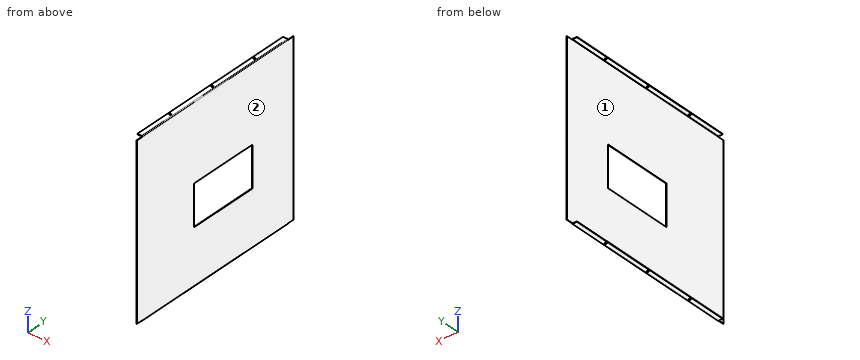
```python
from build123d import *

# Parameters (mm, degrees)
SKETCH_1_W                       = 1.5
SKETCH_1_H                       = 560.17
SM_BASE_FLANGE_1_DEPTH           = 500
SKETCH_6_W                       = 317.570371398
SKETCH_6_H                       = 336.908787646
CUT_EXTRUDE_1_DEPTH              = 10
SKETCH_7_W                       = 1.5
SKETCH_7_H                       = 317.570371398
EXTRUDE_1_DEPTH                  = 34.77
SKETCH_8_W                       = 1.5
SKETCH_8_H                       = 317.570371398
EXTRUDE_2_DEPTH                  = 92.14
SKETCH_9_W                       = 1.5
SKETCH_9_H                       = 209.998787646
EXTRUDE_3_DEPTH                  = 126
SKETCH_10_W                      = 1.5
SKETCH_10_H                      = 209.998787646
EXTRUDE_4_DEPTH                  = 73
SM_EDGE_FLANGE_1_STRIP_W         = 7.4732
SM_EDGE_FLANGE_1_STRIP_H         = 1.5
SM_EDGE_FLANGE_1_STRIP_CUT_DEPTH = 560.17
SM_EDGE_FLANGE_1_DEPTH           = 560.17
SM_EDGE_FLANGE_2_STRIP_W         = 7.4732
SM_EDGE_FLANGE_2_STRIP_H         = 1.5
SM_EDGE_FLANGE_2_STRIP_CUT_DEPTH = 560.17
SM_EDGE_FLANGE_2_DEPTH           = 560.17
SKETCH_19_W                      = 22.446307896
SKETCH_19_H                      = 4.345643328
SKETCH_19_H_2                    = 10.457116237
CUT_EXTRUDE_2_DEPTH              = 20
SKETCH_20_W                      = 19.209439619
SKETCH_20_H                      = 11.495536561
SKETCH_20_W_2                    = 27.208670792
SKETCH_20_H_2                    = 7.195465163
CUT_EXTRUDE_3_DEPTH              = 20
SKETCH_21_R                      = 2.75
CUT_EXTRUDE_4_DEPTH              = 20
CUT_EXTRUDE_START                = -10
SKETCH_22_R                      = 2.75
CUT_EXTRUDE_5_DEPTH              = 10


# Sheet-metal steps are written as plain solids
with BuildPart() as part:
    # Sketch 1 → 基体-法兰1 (new body)
    with BuildSketch(Plane.XY):
        with Locations((0.75, 280.085)):
            Rectangle(SKETCH_1_W, SKETCH_1_H)
    extrude(amount=SM_BASE_FLANGE_1_DEPTH)

    # 草图6 → 切除-拉伸1 (cut)
    with BuildSketch(Plane(origin=(1.5, 0, 0), x_dir=(0, 0, -1), z_dir=(1, 0, 0))):
        with Locations((-246.249491055, 280.085)):
            Rectangle(SKETCH_6_W, SKETCH_6_H)
    extrude(amount=-CUT_EXTRUDE_1_DEPTH, mode=Mode.SUBTRACT)

    # 草图7 → 凸台-拉伸1 (add)
    with BuildSketch(Plane.XZ.offset(-448.539393823)):
        with Locations((0.75, 246.249491055)):
            Rectangle(SKETCH_7_W, SKETCH_7_H)
    extrude(amount=EXTRUDE_1_DEPTH)

    # 草图8 → 凸台-拉伸2 (add)
    with BuildSketch(Plane(origin=(0, 111.630606177, 0), x_dir=(1, 0, 0), z_dir=(0, 1, 0))):
        with Locations((0.75, -246.249491055)):
            Rectangle(SKETCH_8_W, SKETCH_8_H)
    extrude(amount=EXTRUDE_2_DEPTH)

    # 草图9 → 凸台-拉伸3 (add)
    with BuildSketch(Plane(origin=(0, 0, 405.034676754), x_dir=(-1, 0, 0), z_dir=(0, 0, -1))):
        with Locations((-0.75, 308.77)):
            Rectangle(SKETCH_9_W, SKETCH_9_H)
    extrude(amount=EXTRUDE_3_DEPTH)

    # 草图10 → 凸台-拉伸4 (add)
    with BuildSketch(Plane.XY.offset(87.464305356)):
        with Locations((0.75, 308.77)):
            Rectangle(SKETCH_10_W, SKETCH_10_H)
    extrude(amount=EXTRUDE_4_DEPTH)

    # 边线-法兰1 strip (across the edge) → 边线-法兰1 strip cut (cut)
    with BuildSketch(Plane(origin=(0, 0, 500), x_dir=(0, 0, -1), z_dir=(0, 1, 0))):
        with Locations((-1.5, -0.75)):
            Rectangle(SM_EDGE_FLANGE_1_STRIP_W, SM_EDGE_FLANGE_1_STRIP_H)
    extrude(amount=SM_EDGE_FLANGE_1_STRIP_CUT_DEPTH, mode=Mode.SUBTRACT)

    # 边线-法兰1 section (across the edge) → 边线-法兰1 (add)
    with BuildSketch(Plane(origin=(0, 0, 500), x_dir=(0, 0, -1), z_dir=(0, 1, 0))):
        with BuildLine():
            Line((0, 0.7366), (0, 13.5))
            Line((0, 13.5), (1.5, 13.5))
            Line((1.5, 13.5), (1.5, 0.7366))
            ThreePointArc((1.5, 0.7366), (1.715745145, 0.215745145), (2.2366, 0))
            Line((2.2366, 0), (2.2366, -1.5))
            ThreePointArc((2.2366, -1.5), (0.655084973, -0.844915027), (0, 0.7366))
        make_face()
    extrude(amount=SM_EDGE_FLANGE_1_DEPTH)

    # 边线-法兰2 strip (across the edge) → 边线-法兰2 strip cut (cut)
    with BuildSketch(Plane(origin=(0, 560.17, 0), x_dir=(0, 0, 1), z_dir=(0, -1, 0))):
        with Locations((-1.5, -0.75)):
            Rectangle(SM_EDGE_FLANGE_2_STRIP_W, SM_EDGE_FLANGE_2_STRIP_H)
    extrude(amount=SM_EDGE_FLANGE_2_STRIP_CUT_DEPTH, mode=Mode.SUBTRACT)

    # 边线-法兰2 section (across the edge) → 边线-法兰2 (add)
    with BuildSketch(Plane(origin=(0, 560.17, 0), x_dir=(0, 0, 1), z_dir=(0, -1, 0))):
        with BuildLine():
            Line((0, 0.7366), (0, 13.5))
            Line((0, 13.5), (1.5, 13.5))
            Line((1.5, 13.5), (1.5, 0.7366))
            ThreePointArc((1.5, 0.7366), (1.715745145, 0.215745145), (2.2366, 0))
            Line((2.2366, 0), (2.2366, -1.5))
            ThreePointArc((2.2366, -1.5), (0.655084973, -0.844915027), (0, 0.7366))
        make_face()
    extrude(amount=SM_EDGE_FLANGE_2_DEPTH)

    # 草图19 → 切除-拉伸2 (cut)
    with BuildSketch(Plane.XZ):
        with Locations((-9.723153948, 0.063778336)):
            Rectangle(SKETCH_19_W, SKETCH_19_H)
        with Locations((-9.723153948, 502.991958119)):
            Rectangle(SKETCH_19_W, SKETCH_19_H_2)
    extrude(amount=-CUT_EXTRUDE_2_DEPTH, mode=Mode.SUBTRACT)

    # 草图20 → 切除-拉伸3 (cut)
    with BuildSketch(Plane(origin=(0, 560.17, 0), x_dir=(1, 0, 0), z_dir=(0, 1, 0))):
        with Locations((-8.10471981, -503.511168281)):
            Rectangle(SKETCH_20_W, SKETCH_20_H)
        with Locations((-12.104335396, 1.361132582)):
            Rectangle(SKETCH_20_W_2, SKETCH_20_H_2)
    extrude(amount=-CUT_EXTRUDE_3_DEPTH, mode=Mode.SUBTRACT)

    # 草图21 → 切除-拉伸4 (cut)
    with BuildSketch(Plane.XY.offset(1.5)):
        with Locations((-7.1183, 430.085)):
            Circle(SKETCH_21_R)
        with Locations((-7.1183, 280.085)):
            Circle(SKETCH_21_R)
        with Locations(Location((-7.1183, 130.085, 0), (0, 0, 180))):
            Circle(SKETCH_21_R)
    extrude(amount=-CUT_EXTRUDE_4_DEPTH, mode=Mode.SUBTRACT)

    # 草图22 → 切除-拉伸5 (cut)
    with BuildSketch(Plane(origin=(0, 0, 498.5), x_dir=(-1, 0, 0), z_dir=(0, 0, -1)).offset(CUT_EXTRUDE_START)):
        with Locations(Location((7.1183, 430.085, 0), (0, 0, 180))):
            Circle(SKETCH_22_R)
        with Locations(Location((7.1183, 280.085, 0), (0, 0, 180))):
            Circle(SKETCH_22_R)
        with Locations((7.1183, 130.085)):
            Circle(SKETCH_22_R)
    extrude(amount=CUT_EXTRUDE_5_DEPTH, mode=Mode.SUBTRACT)


solid = part.part
```
The listing builds one solid part. Answer for the finished solid, in the listing's coordinates (mm). Face numbers are marked on the shaded views. Round coordinates to 2 decimals unless told otherwise and drop trailing zeros. Order: outer loops, then holes, each group sorted by start corner. A loop starts at its lowest first (then second) coordinate and runs counter-clockwise, first axis right, second up. Notation, with made-up numbers: (-20.75, 74.25) - (22.25, 74.25) arc R29 ccw to (22.25, 105.25) - close; hole circle Ø10 at (-25.75, 78.5). An arc over 180 degrees is marked (long way). Put each result on its own line as item: value. Start each with the question number.
(1) Given P1, Ø0.8, axis at x = 0.5, y = 554, coming from the +Z side; P2, Ø2.5, axis at x = -9, z = 499, coming from the -Y side; P3, Ø6.5, axis at x = -8.5, y = 316.5, coming from the -Z side; P4, Ø1, axis at y = 117, z = 303, coming from the -X side, each flat-ended and moving along its own axis, determine where each tip first touches the part or whether it passes through.
(2) Straight lines are drawn through the part: probe 1 along Z at (x, y) = (-11.75, 299); probe 2 along X at (y, z) = (148.5, 446). For each, find the intervals that lie inside material, in ascending order. Write a range as from..to.
(3) Find section D-D (z = 342). Give the vertices of the cut face in (x, y), plus the area to 3 significant figures.
(4) Find section B-B (y = 265). Give the vertices of the cut face in (x, z), plus the area to 3 significant figures.
(5) Find section A-A (z = 230). Give the vertices of the cut face in (x, y).
(6) Find section C-C (y = 511.5). Give the vertices of the cut face in (x, z).
(7) Determine the mould class of the marked faces 1 and 2 for opening direction Z: released by +Z, released by -Z, zero draft, split by the parting line, or undercut.
Reply:
1. P1: z = 497.76
1. P2: y = 20
1. P3: z = 0
1. P4: x = 0
2. probe 1: 0..1.5, 498.5..500
2. probe 2: 0..1.5
3. outline: (0, 0) - (1.5, 0) - (1.5, 560.17) - (0, 560.17) - close
3. area: 840 mm^2
4. outline: (-13.5, 0) - (-0.74, 0) arc R2.24 ccw to (1.5, 2.24) - (1.5, 160.46) - (0, 160.46) - (0, 2.24) arc R0.74 cw to (-0.74, 1.5) - (-13.5, 1.5) - close; (-13.5, 498.5) - (-0.74, 498.5) arc R0.74 cw to (0, 497.76) - (0, 279.03) - (1.5, 279.03) - (1.5, 497.76) arc R2.24 ccw to (-0.74, 500) - (-13.5, 500) - close
4. area: 611 mm^2
5. outline: (0, 0) - (1.5, 0) - (1.5, 203.77) - (0, 203.77) - close; (0, 413.77) - (1.5, 413.77) - (1.5, 560.17) - (0, 560.17) - close
6. outline: (-13.5, 0) - (-0.74, 0) arc R2.24 ccw to (1.5, 2.24) - (1.5, 497.76) arc R2.24 ccw to (-0.74, 500) - (-13.5, 500) - (-13.5, 498.5) - (-0.74, 498.5) arc R0.74 cw to (0, 497.76) - (0, 2.24) arc R0.74 cw to (-0.74, 1.5) - (-13.5, 1.5) - close
7. face 1: undercut
7. face 2: zero draft
